```python
from build123d import *

# Parameters (mm, degrees)
BOSS_EXTRUDE1_DEPTH      = 127
SKETCH2_R                = 78.74
BOSS_EXTRUDE2_DEPTH      = 127
BOSS_EXTRUDE3_DEPTH      = 40.132
SKETCH4_W                = 50.8
SKETCH4_H                = 127
BOSS_EXTRUDE4_DEPTH      = 127
CUT_EXTRUDE1_DEPTH       = 643.951973118
BOSS_EXTRUDE6_DEPTH      = 63.5
BOSS_EXTRUDE7_DEPTH      = 0.254
SKETCH10_R               = 78.74
BOSS_EXTRUDE8_DEPTH      = 127
CUT_EXTRUDE4_DEPTH       = 1270
SKETCH12_R               = 38.1
BOSS_EXTRUDE9_DEPTH      = 152.4
SKETCH13_R               = 25.4
BOSS_EXTRUDE10_DEPTH     = 50.8
BOSS_EXTRUDE11_DEPTH     = 127
CUT_EXTRUDE16_DEPTH      = 0.508
CUT_EXTRUDE17_REACH      = 733.584
CUT_EXTRUDE17_END_RADIUS = 78.74
SKETCH25_W               = 132.08
SKETCH25_H               = 81.28
SKETCH25_R               = 31.75
SKETCH26_R               = 25.4
CUT_EXTRUDE18_DEPTH      = 76.2


with BuildPart() as part:
    # Sketch1 → Boss-Extrude1 (new body)
    with BuildSketch(Plane(origin=(0, 0, 0), x_dir=(1, 0, 0), z_dir=(0, 1, 0))):
        with BuildLine():
            Line((0, 0), (76.2, 0))
            Line((76.2, 0), (101.6, 0))
            ThreePointArc((101.6, 0), (191.402561211, 37.197438789), (228.6, 127))
            Line((228.6, 127), (228.6, 326.115224022))
            ThreePointArc((228.6, 326.115224022), (206.586135695, 398.822078741), (147.938986841, 447.106743761))
            Line((147.938986841, 447.106743761), (123.740682893, 457.189370406))
            Line((123.740682893, 457.189370406), (3.117633302, 457.189370406))
            Line((3.117633302, 457.189370406), (3.117633302, 507.989370406))
            Line((3.117633302, 507.989370406), (130.117633302, 507.989370406))
            Line((130.117633302, 507.989370406), (180.917633302, 507.989370406))
            add(Edge.make_bspline(
                [(180.917633302, 507.989370406), (258.096842752, 507.989370406), (279.4, 408.366132146), (279.4, 351.515224022)],
                knots=[0, 0, 0, 0, 0.284383622, 0.284383622, 0.284383622, 0.284383622], degree=3))
            Line((279.4, 351.515224022), (279.4, 97.515224022))
            add(Edge.make_bspline(
                [(279.4, 97.515224022), (279.4, 39.949501281), (253.612703292, -50.8), (177.8, -50.8)],
                knots=[0.713423735, 0.713423735, 0.713423735, 0.713423735, 1, 1, 1, 1], degree=3))
            Line((177.8, -50.8), (127, -50.8))
            Line((127, -50.8), (0, -50.8))
            Line((0, -50.8), (0, 0))
        make_face()
    extrude(amount=BOSS_EXTRUDE1_DEPTH)

    # Sketch2 → Boss-Extrude2 (add)
    with BuildSketch(Plane.ZY.offset(-3.117633302)):
        with Locations((-482.589370406, 63.5)):
            Circle(SKETCH2_R)
    extrude(amount=BOSS_EXTRUDE2_DEPTH)

    # Sketch3 → Boss-Extrude3 (add)
    with BuildSketch(Plane.ZY.offset(123.882366698)):
        Polygon((-435.664699602, 63.970535124), (-459.534530374, 104.373224542), (-506.459201178, 103.902689418), (-529.514041209, 63.029464876), (-505.644210437, 22.626775458), (-458.719539633, 23.097310582), align=None)
    extrude(amount=BOSS_EXTRUDE3_DEPTH)

    # Sketch4 → Boss-Extrude4 (add)
    with BuildSketch(Plane.ZY):
        with Locations((25.4, 63.5)):
            Rectangle(SKETCH4_W, SKETCH4_H)
    extrude(amount=BOSS_EXTRUDE4_DEPTH)

    # Sketch5 → Cut-Extrude1 (cut, through all)
    with BuildSketch(Plane(origin=(0, 0, 0), x_dir=(-1, 0, 0), z_dir=(0, -1, 0))):
        Polygon((127, -38.1), (127, 0), (-25.4, 0), align=None)
    extrude(amount=-CUT_EXTRUDE1_DEPTH, mode=Mode.SUBTRACT)

    # Sketch7 → Boss-Extrude6 (add)
    with BuildSketch(Plane.XY.offset(50.8)):
        Polygon((-60.382366698, 110.42702988), (-101.022366698, 86.96351494), (-101.022366698, 40.03648506), (-60.382366698, 16.57297012), (-19.742366698, 40.03648506), (-19.742366698, 86.96351494), align=None)
    extrude(amount=-BOSS_EXTRUDE6_DEPTH)

    # Sketch9 → Boss-Extrude7 (add)
    with BuildSketch(Plane.XY.offset(50.8)):
        Polygon((-61.941183349, 110.42702988), (-102.581183349, 86.96351494), (-102.581183349, 40.03648506), (-61.941183349, 16.57297012), (-21.301183349, 40.03648506), (-21.301183349, 86.96351494), align=None)
    extrude(amount=BOSS_EXTRUDE7_DEPTH)

    # Sketch10 → Boss-Extrude8 (add)
    with BuildSketch(Plane.XY.offset(50.8)):
        with Locations(Location((-61.941183349, 63.970535124, 0), (0, 0, 145.715287544))):
            Circle(SKETCH10_R)
    extrude(amount=BOSS_EXTRUDE8_DEPTH)

    # Sketch11 → Cut-Extrude4 (cut, symmetric)
    with BuildSketch(Plane(origin=(-139.7, 0, 0), x_dir=(0, 0, -1), z_dir=(1, 0, 0))):
        Polygon((-201.145745502, -18.230355882), (-201.145745502, 206.905410628), (-111.777750152, 206.905410628), (-201.145745502, -183.515968434), align=None)
    extrude(amount=CUT_EXTRUDE4_DEPTH, both=True, mode=Mode.SUBTRACT)

    # Sketch12 → Boss-Extrude9 (add)
    with BuildSketch(Plane.XY.offset(50.8)):
        with Locations(Location((-61.941183349, 63.970535124, 0), (0, 0, 90))):
            Circle(SKETCH12_R)
    extrude(amount=BOSS_EXTRUDE9_DEPTH)

    # Sketch13 → Boss-Extrude10 (add)
    with BuildSketch(Plane.XY.offset(203.2)):
        with Locations((-61.941183349, 63.970535124)):
            Circle(SKETCH13_R)
    extrude(amount=BOSS_EXTRUDE10_DEPTH)

    # Sketch18 → Boss-Extrude11 (add)
    with BuildSketch(Plane(origin=(0, 0, 0), x_dir=(0, 0, -1), z_dir=(1, 0, 0))):
        Polygon((-50.8, -14.769464876), (-90.168883972, -135.51337145), (-162.615227917, -111.892041067), (-123.246343944, 8.851865507), align=None)
    extrude(amount=-BOSS_EXTRUDE11_DEPTH)

    # Sketch24 → Cut-Extrude16 (cut)
    with BuildSketch(Plane(origin=(0, 127, 0), x_dir=(1, 0, 0), z_dir=(0, 1, 0))):
        Polygon((20.493010652, -50.8), (20.493010652, -1.226747337), (-127, -38.1), (-127, -50.8), align=None)
    extrude(amount=-CUT_EXTRUDE16_DEPTH, mode=Mode.SUBTRACT)

    # Cut-Extrude17: up to this cylinder (the profile starts outside it)
    cut_extrude17_end = Plane(origin=(-61.941183349, 63.970535124, 126.392056), z_dir=(0, 0, -1)) * Cylinder(CUT_EXTRUDE17_END_RADIUS, 1625.648, mode=Mode.PRIVATE)
    # Sketch25 → Cut-Extrude17 (cut, up to the surface)
    with BuildSketch(Plane(origin=(0, -149.065926338, 48.603356681), x_dir=(1, 0, 0), z_dir=(0, -0.950739421843146, 0.3099912123808683)), mode=Mode.PRIVATE) as cut_extrude17_sk1:
        with Locations((-63.5, 81.819158306)):
            Rectangle(SKETCH25_W, SKETCH25_H)
        with Locations(Location((-63.5, 81.819158306, 0), (0, 0, 270))):
            Circle(SKETCH25_R, mode=Mode.SUBTRACT)
    cut_extrude17_tool1 = extrude(cut_extrude17_sk1.sketch, amount=-CUT_EXTRUDE17_REACH, mode=Mode.PRIVATE) - cut_extrude17_end
    add(cut_extrude17_tool1.solids().sort_by_distance((0.989143, -123.702706, 126.392056))[0], mode=Mode.SUBTRACT)

    # Sketch26 → Cut-Extrude18 (cut)
    with BuildSketch(Plane(origin=(0, -149.065926338, 48.603356681), x_dir=(1, 0, 0), z_dir=(0, -0.950739421843146, 0.30999121238086846))):
        with Locations(Location((-63.5, 81.819158306, 0), (0, 0, 270))):
            Circle(SKETCH26_R)
    extrude(amount=-CUT_EXTRUDE18_DEPTH, mode=Mode.SUBTRACT)


solid = part.part
```
Work out the finished part from the listing and answer in its coordinate system (mm). A direction names the side the tool comes from. Round coordinates to 2 decimals unless told otherwise and drop trailing zeros. Write each loop counter-clockwise with the first axis right and the second up, starting at its lowest first coordinate (ties: lowest second). Pieces come first, ordered by that corner, then holes. Notation, with made-up numbers: (82, 60.25) - (97, 60.25) arc R22 cw to (97, 88.25) - close; hole circle Ø1 at (34.5, -1.75). An arc over 180 degrees is marked (long way). Return JSON: item names as keys, results as strings. Group by question number.
Q1. The part is cut by section B-B on z = -161. Write down the section's boundary in (x, y), then the cut area to 3 significant figures.
Q2. The part is cut by section A-A on x = 87.5. Write down the section's boundary in (y, z).
Q3. Each of these flat-tipped pins is pushed along its axis until it touches: pin 1 Ø5.5 at (y, z) = (7, 39.5) entering from -X; pin 2 Ø24.5 at (x, y) = (-74.5, 82.5) entering from -Z; pin 3 Ø23 at (x, y) = (82.5, 53) entering from -Z. Where does it stop, or does it pass through?
Q4. The mould has two halves that part along X. Classify faces 4 (the flat face through (-37, 72, 203.2)), 5 (the flat face through (279.4, 63, -226)), 6 (the cylindrical face through (207.18, 62.61, -397.92)), 7 (the cylindrical face through (-75.66, -73.796, 79.271)): released by +X, released by -X, zero draft, split by the parting line, or undercut.
Q5. Find the intervals of material crossed by L1, parallel to X at y = -113.5, z = 124; L2, parallel to X at y = 28.5, z = -305; L3, parallel to Y at x = 255, z = -87, in increasing order.
Q6. For faces 1 (the flat face through (-62, -5, 50.8)), 2 (the flat face through (64, 63, 0)), 3 (the flat face through (-143.7, 83.8, -517.8)), determine the directions among +Z, -Z, +X, -X, +Y, -Y from which every point of the face is accessible in a straight line to the end or side of a thin tool.
Solved:
{
 "1": {"outline": "(228.6, 0) - (279.4, 0) - (279.4, 127) - (228.6, 127) - close", "area": "6,450 mm²"},
 "2": {"outline": "(0, -507.99) - (127, -507.99) - (127, -457.19) - (0, -457.19) - close; (0, 0) - (127, 0) - (127, 50.8) - (0, 50.8) - close"},
 "3": {"pin 1": "x = -127", "pin 2": "z = -561.04", "pin 3": "z = -507.99"},
 "4": {"face 4": "zero draft", "face 5": "released by +X", "face 6": "undercut", "face 7": "split by the parting line"},
 "5": {"L1": "-95.24 to -88.88, -38.12 to -31.76", "L2": "228.6 to 279.4", "L3": "0 to 127"},
 "6": {"face 1": "+X, -X, -Y", "face 2": "+Y, -Y", "face 3": "-Z, -X, +Y"}
}
